```python
from build123d import *

# Parameters (mm, degrees)
SKETCH001_W     = 105
SKETCH001_H     = 71
PAD_DEPTH       = 3
SKETCH_W        = 80
SKETCH_H        = 65
POCKET_DEPTH    = 5
SKETCH002_R     = 2
POCKET001_DEPTH = 5
SKETCH003_R     = 2
POCKET002_DEPTH = 5
SKETCH004_R     = 2
POCKET003_DEPTH = 5
SKETCH005_R     = 2
POCKET004_DEPTH = 5
SKETCH006_W     = 15
SKETCH006_H     = 65
PAD001_DEPTH    = 3
SKETCH007_W     = 15
SKETCH007_H     = 30
POCKET005_DEPTH = 3


with BuildPart() as part:
    # Sketch001 → Pad (new body)
    with BuildSketch(Plane.XY):
        with Locations((42.5, 32.5)):
            Rectangle(SKETCH001_W, SKETCH001_H)
    extrude(amount=PAD_DEPTH)

    # Sketch → Pocket (cut)
    with BuildSketch(Plane.XY):
        with Locations((40, 32.5)):
            Rectangle(SKETCH_W, SKETCH_H)
    extrude(amount=POCKET_DEPTH, mode=Mode.SUBTRACT)

    # Sketch002 → Pocket001 (cut)
    with BuildSketch(Plane.XY):
        with Locations((-6, 10)):
            Circle(SKETCH002_R)
    extrude(amount=POCKET001_DEPTH, mode=Mode.SUBTRACT)

    # Sketch003 → Pocket002 (cut)
    with BuildSketch(Plane.XY):
        with Locations((-6, 55)):
            Circle(SKETCH003_R)
    extrude(amount=POCKET002_DEPTH, mode=Mode.SUBTRACT)

    # Sketch004 → Pocket003 (cut)
    with BuildSketch(Plane.XY):
        with Locations((91, 10)):
            Circle(SKETCH004_R)
    extrude(amount=POCKET003_DEPTH, mode=Mode.SUBTRACT)

    # Sketch005 → Pocket004 (cut)
    with BuildSketch(Plane.XY):
        with Locations((91, 55)):
            Circle(SKETCH005_R)
    extrude(amount=POCKET004_DEPTH, mode=Mode.SUBTRACT)

    # Sketch006 → Pad001 (join)
    with BuildSketch(Plane.XY):
        with Locations((7.5, 32.5)):
            Rectangle(SKETCH006_W, SKETCH006_H)
    extrude(amount=PAD001_DEPTH)

    # Sketch007 → Pocket005 (cut)
    with BuildSketch(Plane.XY):
        with Locations((7.5, 35)):
            Rectangle(SKETCH007_W, SKETCH007_H)
    extrude(amount=POCKET005_DEPTH, mode=Mode.SUBTRACT)


solid = part.part
```
The model under review builds one solid part; all positions refer to its coordinate system, in mm. A direction names the side the tool comes from. Coordinates: 2 decimals unless noted, no trailing zeros. Write each loop counter-clockwise with the first axis right and the second up, starting at its lowest first coordinate (ties: lowest second). Pieces come first, ordered by that corner, then holes. Notation, with made-up numbers: (30.5, 42) - (73.5, 42) arc R18 ccw to (73.5, 56) - close; hole circle Ø6 at (7.5, 70). An arc over 180 degrees is marked (long way). Answer in a Markdown table with one row per item. Add a question column.
Q1. Draft analysis for pull direction Y (two halves, no side actions). For faces 3 (the face through (42, -3, 1)), 4 (the face through (42, 68, 1)), 5 (the face through (-10, 32, 1)), 6 (the face through (92.908, 10.601, 1.479)), state which applies: +Y half, -Y half, draft (parallel to the pull), parting line (faces both ways), or undercut.
Q2. Consider section A-A on y = 27. Give the boundary of the cut face in (x, z), then the cut area to 3 significant figures.
Q3. To check wall thickness, follow line 1 along Y through (x, z) = (91, 1.6); line 2 along X through (y, z) = (55, 1.6); line 3 along Y through (x, z) = (29.5, 0.7). State the ranges of each line that lie inside material, in increasing order. Write a range as from..to.
Q4. For faces 1 (the face through (11.1, 19.5, 0)), 2 (the face through (0, 35, 1)), list the 3-axis set-ups (+Z, -Z, +X, -X, +Y, -Y) from which the entire face can be reached by the end or side of a thin tool; tool diameter is ignored.
Q5. Consider section C-C on y = 10. Give the boundary of the cut face in (x, z).
Q6. Consider section B-B on x = 51.5. Give the boundary of the cut face in (y, z), then the cut area to 3 significant figures.
Q7. Consider section D-D on z = 1.6. Give the boundary of the cut face in (x, y).
Q8. Clearance check with a flat-ended pin moving along its axis: pin 1 (3 mm diameter, centred on x = 91, y = 10, fed in from +Z). State where the tip first meets the part, or that it passes through.
Answers below:
| question | item | result |
|---|---|---|
| 1 | face 3 | -Y half |
| 1 | face 4 | +Y half |
| 1 | face 5 | draft |
| 1 | face 6 | undercut |
| 2 | outline | (-10, 0) - (0, 0) - (0, 3) - (-10, 3) - close; (80, 0) - (95, 0) - (95, 3) - (80, 3) - close |
| 2 | area | 75.0 mm² |
| 3 | line 1 | -3..8, 12..53, 57..68 |
| 3 | line 2 | -10..-8, -4..15, 80..89, 93..95 |
| 3 | line 3 | -3..0, 65..68 |
| 4 | face 1 | -Z, +X, -X, +Y, -Y |
| 4 | face 2 | +Z, -Z |
| 5 | outline | (-10, 0) - (-8, 0) - (-8, 3) - (-10, 3) - close; (-4, 0) - (15, 0) - (15, 3) - (-4, 3) - close; (80, 0) - (89, 0) - (89, 3) - (80, 3) - close; (93, 0) - (95, 0) - (95, 3) - (93, 3) - close |
| 6 | outline | (-3, 0) - (0, 0) - (0, 3) - (-3, 3) - close; (65, 0) - (68, 0) - (68, 3) - (65, 3) - close |
| 6 | area | 18.0 mm² |
| 7 | outline | (-10, -3) - (95, -3) - (95, 68) - (-10, 68) - close; hole circle Ø4 at (-6, 10); hole circle Ø4 at (-6, 55); hole (0, 20) - (15, 20) - (15, 0) - (80, 0) - (80, 65) - (15, 65) - (15, 50) - (0, 50) - close; hole circle Ø4 at (91, 10); hole circle Ø4 at (91, 55) |
| 8 | pin 1 | through |
